Geometry: final body of the model. Coordinates: model frame, mm. A direction names the side the tool comes from. Give positions to 0.01 mm unless a question says otherwise; leave off trailing zeros. Write each loop counter-clockwise with the first axis right and the second up, starting at its lowest first coordinate (ties: lowest second). Pieces come first, ordered by that corner, then holes. Notation, with made-up numbers: M -36.5,-0.75 L -7.5,-0.75 A12 ccw -7.5,18.25 Z; hole C -18,3 d11. An arc over 180 degrees is marked long. Use a Markdown table: item, result. Add a question column.
1) Section A-A on x = 675. Return the cut outline in (y, z).
2) Set-up query: faces 1 (the flat face through (672, -725, 215)), 2 (the flat face through (875, -237, 116)), 3 (the flat face through (50, -62, 30)). Return all of +Z, -Z, +X, -X, +Y, -Y with unobstructed straight access to the full face (end or side cutting, diameter ignored); none if empty.
3) Section B-B on z = 69. Return the cut outline in (x, y), then the cut area to 3 significant figures.
4) Draft query along Y for faces 4 (the flat face through (548, -225, 174)), 5 (the flat face through (548, -50, 174)), 6 (the cylindrical face through (678.199, -712.325, 414.973)). Return one class per face: +Y half, -Y half, draft (parallel to the pull), parting line (faces both ways), or undercut.
5) Pin query (flat end, axial travel): pin 1 (12.5 mm diameter, centred on y = -706.5, z = 129, fed in from +X); pin 2 (3 mm diameter, centred on y = -450.5, z = 159, fed in from -X); pin 3 (20 mm diameter, centred on y = -232.5, z = 22, fed in from -X); pin 4 (1 mm diameter, centred on x = 311.5, y = -580.5, fed in from -Z). Return the tip coordinate at first contact, or that it passes through.
6) Line query: line 1 (Y direction, x = 607.5, z = 146.5); line 2 (Y direction, x = 441, z = 307); line 3 (Z direction, x = 602, y = -500). Output: solid intervals per line, ascending.
7) Section C-C on y = -375. Return the cut outline in (x, z), then the cut area to 3 significant figures.
8) Section D-D on x = 528. Return the cut outline in (y, z), then the cut area to 3 significant figures.
```python
from build123d import *

# Parameters (mm, degrees)
F4_DEPTH  = 10
F5_DEPTH  = 25
F8_DEPTH  = 25
F9_R      = 87.5
F10_DEPTH = 650


with BuildPart() as f4:
    # F0 (on Top) → F4 (new body)
    with BuildSketch(Plane.XY):
        Polygon((900, 0), (0, 0), (0, -500), (400, -800), (900, -800), align=None)
    extrude(amount=F4_DEPTH)

    # F3 (on offset) → F8 (join)
    with BuildSketch(Plane.XZ.offset(700)):
        with BuildLine():
            Line((864.9955457431, 0), (864.9955457431, 223.6990012303))
            ThreePointArc((864.9955457431, 223.6990012303), (673.9888114785, 414.9973091856), (485.0290649374, 221.6767739387))
            Line((485.0290649374, 221.6767739387), (485.0290649374, 0))
            Line((485.0290649374, 0), (864.9955457431, 0))
        make_face()
    extrude(amount=F8_DEPTH)



with BuildPart() as f5:
    # F1 (on Front) → F5 (new body)
    with BuildSketch(Plane.XZ):
        with BuildLine():
            Line((50, 50), (50, 0))
            Line((50, 0), (875, 0))
            Line((875, 0), (875, 225))
            ThreePointArc((875, 225), (769.5256396076, 401.2523856768), (564.3509654323, 391.6036948847))
            Line((564.3509654323, 391.6036948847), (50, 50))
        make_face()
    extrude(amount=F5_DEPTH)


with BuildPart() as f5_1:
    # F6: moved
    add(f5.part.moved(Location((0, -50, 0))))


with BuildPart() as f7_1:
    # F7: copy of F5
    add(f5_1.part.moved(Location((0, -175, 0))))


with BuildPart() as f4_1:
    add(f4.part)

    add(f5_1.part)  # F10 merges F5

    add(f7_1.part)  # F10 merges F7_1
    # F9 (on offset) → F10 (join, through all)
    with BuildSketch(Plane.XZ.offset(700)):
        with Locations((675, 225)):
            Circle(F9_R)
    extrude(amount=-F10_DEPTH)


solid = f4_1.part
```
Found:
| question | item | result |
|---|---|---|
| 1 | outline | M -800,0 L 0,0 L 0,10 L -50,10 L -50,425 L -75,425 L -75,312.5 L -225,312.5 L -225,425 L -250,425 L -250,312.5 L -700,312.5 L -700,415 L -725,415 L -725,10 L -800,10 Z; hole M -700,10 L -250,10 L -250,137.5 L -700,137.5 Z; hole M -225,10 L -75,10 L -75,137.5 L -225,137.5 Z |
| 2 | face 1 | +Z, +X, -X, -Y |
| 2 | face 2 | +Z, +X, +Y, -Y |
| 2 | face 3 | +Z, -X, +Y, -Y |
| 3 | outline | M 78.61,-250 L 875,-250 L 875,-225 L 78.61,-225 Z; M 78.61,-75 L 875,-75 L 875,-50 L 78.61,-50 Z; M 485.03,-725 L 865,-725 L 865,-700 L 485.03,-700 Z |
| 3 | area | 49,300 mm² |
| 4 | face 4 | undercut |
| 4 | face 5 | +Y half |
| 4 | face 6 | draft |
| 5 | pin 1 | x = 865 |
| 5 | pin 2 | x = 615.87 |
| 5 | pin 3 | x = 50 |
| 5 | pin 4 | z = 0 |
| 6 | line 1 | -725 to -700, -250 to -225, -75 to -50 |
| 6 | line 2 | -250 to -225, -75 to -50 |
| 6 | line 3 | 0 to 10, 176.76 to 273.24 |
| 7 | outline | M 0,0 L 900,0 L 900,10 L 0,10 Z; C 675,225 d175 |
| 7 | area | 33,100 mm² |
| 8 | outline | M -800,0 L 0,0 L 0,10 L -50,10 L -50,367.46 L -75,367.46 L -75,10 L -225,10 L -225,367.46 L -250,367.46 L -250,10 L -700,10 L -700,345.38 L -725,345.38 L -725,10 L -800,10 Z |
| 8 | area | 34,300 mm² |
